Could you check a few things on this model? Use its own coordinates, in mm. Face numbers are marked on the shaded views. A direction names the side the tool comes from. Give positions to 0.01 mm unless a question says otherwise; leave off trailing zeros. Order: outer loops, then holes, each group sorted by start corner. A loop starts at its lowest first (then second) coordinate and runs counter-clockwise, first axis right, second up. Notation, with made-up numbers: M 56.25,55 L 61.25,55 A8 ccw 61.25,70 Z; hole C -31,89 d2. An arc over 180 degrees is marked long. Use a Markdown table: item, result. Add a question column.
Item 1: Suppose I cut it at C-C on y = 10. Count the separate pieces of the cut face and the enclosed holes in it, plus the area to 3 significant figures.
Item 2: If we mould it in two halves opening along X, with no side actions, what happens to the marked faces 1, 2, 3 and 4? For each: released by +X, released by -X, zero draft, split by the parting line, or undercut.
Item 3: For the marked faces 5, 6 and 7, which set-ups out of +Z, -Z, +X, -X, +Y, -Y let a thin tool reach every point of the face, with its end or its side?
Item 4: Suppose I cut it at D-D on z = 14. Write out the boundary of the cut face in (x, y).
Item 5: I'm going to push flat-ended pins straight in: pin 1 Ø10 at (x, y) = (12, 8.5) entering from +Z; pin 2 Ø1 at (y, z) = (8.5, 18) entering from +X; pin 3 Ø4 at (x, y) = (65, 10) entering from -Z; pin 4 Ø7.5 at (x, y) = (65, 10) entering from +Z. Where does each tip first touch, or does it pass through?
Item 6: If I drill on L1, parallel to Y at x = 5, z = 4; L2, parallel to X at y = 14.75, z = 12.75; L3, parallel to Y at x = 65, z = 13.75, over which ranges is the centre line in solid material (lowest first)? Write a range as from..to.
Item 7: Suppose I cut it at B-B on x = 35. Write out the boundary of the cut face in (y, z).
Item 8: Suppose I cut it at A-A on z = 5.5. Write out the boundary of the cut face in (x, y), plus the area to 3 significant figures.
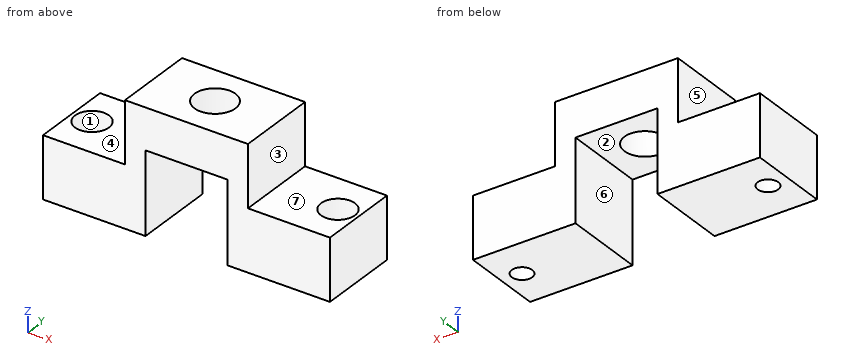
from build123d import *

# Parameters (mm, degrees)
SKETCH1_W           = 70
SKETCH1_H           = 20
SKETCH1_R           = 2.5
BOSS_EXTRUDE1_DEPTH = 15
SKETCH2_W           = 30
SKETCH2_H           = 20
BOSS_EXTRUDE2_DEPTH = 15
SKETCH4_W           = 20
SKETCH4_H           = 20
CUT_EXTRUDE1_DEPTH  = 79.74007874
SKETCH5_R           = 5
CUT_EXTRUDE2_DEPTH  = 79.74007874
SKETCH6_R           = 4.15
CUT_EXTRUDE3_DEPTH  = 5
SKETCH7_R           = 4.15
CUT_EXTRUDE4_DEPTH  = 5


with BuildPart() as part:
    # Sketch1 → Boss-Extrude1 (new body)
    with BuildSketch(Plane.XY):
        with Locations((35, 10)):
            Rectangle(SKETCH1_W, SKETCH1_H)
        with Locations((65, 10)):
            Circle(SKETCH1_R, mode=Mode.SUBTRACT)
        with Locations((5, 10)):
            Circle(SKETCH1_R, mode=Mode.SUBTRACT)
    extrude(amount=BOSS_EXTRUDE1_DEPTH)

    # Sketch2 → Boss-Extrude2 (add)
    with BuildSketch(Plane.XY.offset(15)):
        with Locations((35, 10)):
            Rectangle(SKETCH2_W, SKETCH2_H)
    extrude(amount=BOSS_EXTRUDE2_DEPTH)

    # Sketch4 → Cut-Extrude1 (cut, through all)
    with BuildSketch(Plane(origin=(0, 20, 0), x_dir=(1, 0, 0), z_dir=(0, 1, 0))):
        with Locations((35, -10)):
            Rectangle(SKETCH4_W, SKETCH4_H)
    extrude(amount=-CUT_EXTRUDE1_DEPTH, mode=Mode.SUBTRACT)

    # Sketch5 → Cut-Extrude2 (cut, through all)
    with BuildSketch(Plane.XY.offset(30)):
        with Locations((35, 10)):
            Circle(SKETCH5_R)
    extrude(amount=-CUT_EXTRUDE2_DEPTH, mode=Mode.SUBTRACT)

    # Sketch6 → Cut-Extrude3 (cut)
    with BuildSketch(Plane.XY.offset(15)):
        with Locations((5, 10)):
            Circle(SKETCH6_R)
    extrude(amount=-CUT_EXTRUDE3_DEPTH, mode=Mode.SUBTRACT)

    # Sketch7 → Cut-Extrude4 (cut)
    with BuildSketch(Plane.XY.offset(15)):
        with Locations((65, 10)):
            Circle(SKETCH7_R)
    extrude(amount=-CUT_EXTRUDE4_DEPTH, mode=Mode.SUBTRACT)


solid = part.part
Findings below:
| question | item | result |
|---|---|---|
| 1 | separate pieces | 4 |
| 1 | enclosed holes | 0 |
| 1 | area | 817 mm^2 |
| 2 | face 1 | undercut |
| 2 | face 2 | undercut |
| 2 | face 3 | released by +X |
| 2 | face 4 | zero draft |
| 3 | face 5 | +Z, -X, +Y, -Y |
| 3 | face 6 | -Z, +Y, -Y |
| 3 | face 7 | +Z, +X, +Y, -Y |
| 4 | outline | M 0,0 L 25,0 L 25,20 L 0,20 Z; M 45,0 L 70,0 L 70,20 L 45,20 Z; hole C 5,10 d8.3; hole C 65,10 d8.3 |
| 5 | pin 1 | stops at z = 15 |
| 5 | pin 2 | stops at x = 50 |
| 5 | pin 3 | passes through |
| 5 | pin 4 | stops at z = 10 |
| 6 | L1 | y = 0..7.5, 12.5..20 |
| 6 | L2 | x = 0..25, 45..70 |
| 6 | L3 | y = 0..5.85, 14.15..20 |
| 7 | outline | M 0,20 L 5,20 L 5,30 L 0,30 Z; M 15,20 L 20,20 L 20,30 L 15,30 Z |
| 8 | outline | M 0,0 L 25,0 L 25,20 L 0,20 Z; M 45,0 L 70,0 L 70,20 L 45,20 Z; hole C 5,10 d5; hole C 65,10 d5 |
| 8 | area | 961 mm^2 |
